```python
from build123d import *

# Parameters (mm, degrees)
SKETCH2_W           = 50
SKETCH2_H           = 50
BOSS_EXTRUDE1_DEPTH = 40
SKETCH4_R           = 3.25
CUT_EXTRUDE1_DEPTH  = 6
CUT_EXTRUDE2_DEPTH  = 34
SKETCH6_W           = 8
SKETCH6_H           = 13
CUT_EXTRUDE3_DEPTH  = 24
CUT_EXTRUDE4_DEPTH  = 7
SKETCH8_W           = 15
SKETCH8_H           = 20
CUT_EXTRUDE5_DEPTH  = 33
SKETCH8_3_W         = 5
SKETCH8_3_H         = 20
CUT_EXTRUDE6_DEPTH  = 24
CUT_EXTRUDE7_DEPTH  = 24
SKETCH7_W           = 3
SKETCH7_H           = 2
CUT_EXTRUDE8_DEPTH  = 10
SKETCH9_W           = 3
SKETCH9_H           = 3
CUT_EXTRUDE9_DEPTH  = 10
SKETCH12_W          = 50
SKETCH12_H          = 50
CUT_EXTRUDE10_DEPTH = 5
SKETCH16_W          = 5
SKETCH16_H          = 20
CUT_EXTRUDE11_DEPTH = 4
CUT_EXTRUDE12_DEPTH = 5
CUT_EXTRUDE13_DEPTH = 4
CUT_EXTRUDE14_DEPTH = 4
SKETCH11_W          = 5
SKETCH11_H          = 10
CUT_EXTRUDE15_DEPTH = 5
SKETCH20_R          = 6.5
CUT_EXTRUDE16_DEPTH = 29


with BuildPart() as part:
    # Sketch2 → Boss-Extrude1 (new body)
    with BuildSketch(Plane(origin=(0, 0, 0), x_dir=(1, 0, 0), z_dir=(0, 1, 0))):
        Rectangle(SKETCH2_W, SKETCH2_H)
    extrude(amount=-BOSS_EXTRUDE1_DEPTH)

    # Sketch4 → Cut-Extrude1 (cut)
    with BuildSketch(Plane(origin=(0, 0, 0), x_dir=(1, 0, 0), z_dir=(0, 1, 0))):
        with Locations(Location((15, -12.5, 0), (0, 0, 270))):
            Circle(SKETCH4_R)
        with Locations(Location((-15, -12.5, 0), (0, 0, 270))):
            Circle(SKETCH4_R)
        with Locations(Location((0, -12.5, 0), (0, 0, 270))):
            Circle(SKETCH4_R)
    extrude(amount=-CUT_EXTRUDE1_DEPTH, mode=Mode.SUBTRACT)

    # Sketch5 → Cut-Extrude2 (cut)
    with BuildSketch(Plane.XZ.offset(40)):
        Polygon((19, 12.5), (15, 12.5), (11, 12.5), (11, 6), (19, 6), align=None)
        Polygon((11, 12.5), (15, 12.5), (19, 12.5), (19, 19), (11, 19), align=None)
        Polygon((-11, 12.5), (-15, 12.5), (-19, 12.5), (-19, 6), (-11, 6), align=None)
        Polygon((-19, 12.5), (-15, 12.5), (-11, 12.5), (-11, 19), (-19, 19), align=None)
        Polygon((4, 12.5), (4, 6), (-4, 6), (-4, 19), (4, 19), align=None)
    extrude(amount=-CUT_EXTRUDE2_DEPTH, mode=Mode.SUBTRACT)

    # Sketch6 → Cut-Extrude3 (cut)
    with BuildSketch(Plane.XZ.offset(40)):
        Polygon((-20, 20), (-20, 3), (0, 3), (20, 3), (20, 20), align=None)
        with Locations((-15, 12.5)):
            Rectangle(SKETCH6_W, SKETCH6_H, mode=Mode.SUBTRACT)
        Polygon((4, 6), (0, 6), (-4, 6), (-4, 19), (4, 19), align=None, mode=Mode.SUBTRACT)
        with Locations((15, 12.5)):
            Rectangle(SKETCH6_W, SKETCH6_H, mode=Mode.SUBTRACT)
    extrude(amount=-CUT_EXTRUDE3_DEPTH, mode=Mode.SUBTRACT)

    # Sketch3 → Cut-Extrude4 (cut)
    with BuildSketch(Plane(origin=(0, 0, 0), x_dir=(1, 0, 0), z_dir=(0, 1, 0))):
        Polygon((19.5, 20), (19.5, 0), (-19.5, 0), (-19.5, 20), (0, 20), align=None)
    extrude(amount=-CUT_EXTRUDE4_DEPTH, mode=Mode.SUBTRACT)

    # Sketch8 → Cut-Extrude5 (cut)
    with BuildSketch(Plane.XZ.offset(40)):
        with Locations((-7.5, -10)):
            Rectangle(SKETCH8_W, SKETCH8_H)
        with Locations((7.5, -10)):
            Rectangle(SKETCH8_W, SKETCH8_H)
    extrude(amount=-CUT_EXTRUDE5_DEPTH, mode=Mode.SUBTRACT)

    # Sketch8_3 → Cut-Extrude6 (cut)
    with BuildSketch(Plane.XZ.offset(40)):
        with Locations((-17.5, -10)):
            Rectangle(SKETCH8_3_W, SKETCH8_3_H)
        with Locations((17.5, -10)):
            Rectangle(SKETCH8_3_W, SKETCH8_3_H)
    extrude(amount=-CUT_EXTRUDE6_DEPTH, mode=Mode.SUBTRACT)

    # Sketch8_4 → Cut-Extrude7 (cut)
    with BuildSketch(Plane.XZ.offset(40)):
        Polygon((20, 3), (-20, 3), (-20, 0), (-15, 0), (0, 0), (15, 0), (20, 0), align=None)
    extrude(amount=-CUT_EXTRUDE7_DEPTH, mode=Mode.SUBTRACT)

    # Sketch7 → Cut-Extrude8 (cut)
    with BuildSketch(Plane(origin=(0, -7, 0), x_dir=(1, 0, 0), z_dir=(0, 1, 0))):
        with Locations((-18, 19)):
            Rectangle(SKETCH7_W, SKETCH7_H)
        with Locations((-18, 1)):
            Rectangle(SKETCH7_W, SKETCH7_H)
        with Locations((18, 1)):
            Rectangle(SKETCH7_W, SKETCH7_H)
        with Locations((18, 19)):
            Rectangle(SKETCH7_W, SKETCH7_H)
    extrude(amount=-CUT_EXTRUDE8_DEPTH, mode=Mode.SUBTRACT)

    # Sketch9 → Cut-Extrude9 (cut)
    with BuildSketch(Plane.XZ.offset(40)):
        with Locations((-22.5, 22.5)):
            Rectangle(SKETCH9_W, SKETCH9_H)
        with Locations((-22.5, -22.5)):
            Rectangle(SKETCH9_W, SKETCH9_H)
        with Locations((22.5, -22.5)):
            Rectangle(SKETCH9_W, SKETCH9_H)
        with Locations((22.5, 22.5)):
            Rectangle(SKETCH9_W, SKETCH9_H)
    extrude(amount=-CUT_EXTRUDE9_DEPTH, mode=Mode.SUBTRACT)

    # Sketch12 → Cut-Extrude10 (cut)
    with BuildSketch(Plane.XZ.offset(40)):
        Rectangle(SKETCH12_W, SKETCH12_H)
    extrude(amount=-CUT_EXTRUDE10_DEPTH, mode=Mode.SUBTRACT)

    # Sketch16 → Cut-Extrude11 (cut)
    with BuildSketch(Plane.XZ.offset(16)):
        with Locations((17.5, -10)):
            Rectangle(SKETCH16_W, SKETCH16_H)
        with Locations((-17.5, -10)):
            Rectangle(SKETCH16_W, SKETCH16_H)
    extrude(amount=-CUT_EXTRUDE11_DEPTH, mode=Mode.SUBTRACT)

    # Sketch13 → Cut-Extrude12 (cut)
    with BuildSketch(Plane(origin=(0, 0, -25), x_dir=(-1, 0, 0), z_dir=(0, 0, -1))):
        Polygon((0, -16.279858657), (10, -16.279858657), (10, -22.279858657), (-10, -22.279858657), (-10, -16.279858657), align=None)
    extrude(amount=-CUT_EXTRUDE12_DEPTH, mode=Mode.SUBTRACT)

    # Sketch14 → Cut-Extrude13 (cut)
    with BuildSketch(Plane.XY.offset(-20)):
        Polygon((10, -19.279858657), (10, -12.279858657), (-20, -12.279858657), (-20, -36.279858657), (10, -36.279858657), align=None)
    extrude(amount=-CUT_EXTRUDE13_DEPTH, mode=Mode.SUBTRACT)

    # Sketch18 → Cut-Extrude14 (cut)
    with BuildSketch(Plane(origin=(-20, 0, 0), x_dir=(0, 0, -1), z_dir=(1, 0, 0))):
        Polygon((4, -29), (24, -29), (24, -12.279858657), (20, -12.279858657), (4, -12.279858657), align=None)
    extrude(amount=-CUT_EXTRUDE14_DEPTH, mode=Mode.SUBTRACT)

    # Sketch11 → Cut-Extrude15 (cut)
    with BuildSketch(Plane.XY.offset(25)):
        with Locations((2.5, -28.5)):
            Rectangle(SKETCH11_W, SKETCH11_H)
        with Locations((-2.5, -28.5)):
            Rectangle(SKETCH11_W, SKETCH11_H)
    extrude(amount=-CUT_EXTRUDE15_DEPTH, mode=Mode.SUBTRACT)

    # Sketch20 → Cut-Extrude16 (cut)
    with BuildSketch(Plane.XZ.offset(35)):
        with Locations((0, 12.5)):
            Circle(SKETCH20_R)
        with BuildLine():
            ThreePointArc((-20, 8.346688069), (-12.792059783, 6.38649037), (-8.5, 12.5))
            ThreePointArc((-8.5, 12.5), (-12.792059783, 18.61350963), (-20, 16.653311931))
            Line((-20, 16.653311931), (-20, 8.346688069))
        make_face()
        with BuildLine():
            Line((-20, 8.346688069), (-20, 16.653311931))
            ThreePointArc((-20, 16.653311931), (-21.5, 12.5), (-20, 8.346688069))
        make_face()
        with Locations((15, 12.5)):
            Circle(SKETCH20_R)
    extrude(amount=-CUT_EXTRUDE16_DEPTH, mode=Mode.SUBTRACT)


solid = part.part
```
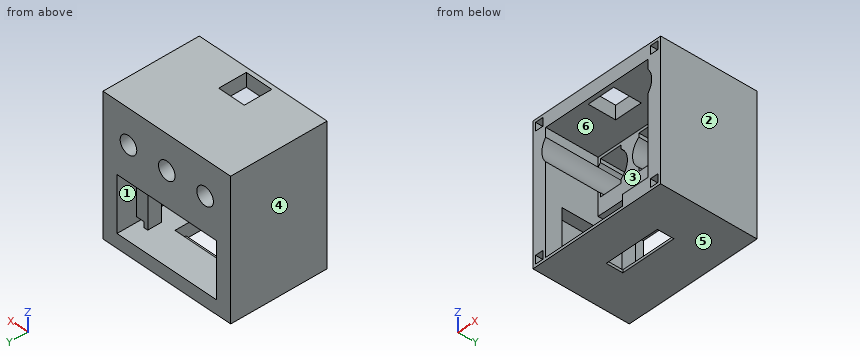
Input: part model. Units: mm. Frame: model coordinates. Face numbers are marked on the shaded views. A direction names the side the tool comes from. Give positions to 0.01 mm unless a question says otherwise; leave off trailing zeros. Order: outer loops, then holes, each group sorted by start corner. A loop starts at its lowest first (then second) coordinate and runs counter-clockwise, first axis right, second up. Notation, with made-up numbers: M 27,73.5 L 32,73.5 A32 ccw 32,107.5 Z; hole C 35,67.25 d6. An arc over 180 degrees is marked long. Return JSON: item names as keys, results as strings.
Item 1: First-contact query: P1, Ø5, axis at x = 15, z = 12.5, coming from the -Y side; P2, Ø12, axis at x = -1.5, z = 8, coming from the -Y side; P3, Ø8.5, axis at x = -15, z = 12.5, coming from the -Y side; P4, Ø10, axis at x = -11, z = -11.5, coming from the +Y side. Flat tips, straight axial feed; report the tip coordinate or a pass-through.
Solutions:
{"P1": "through", "P2": "y = -16", "P3": "y = -6", "P4": "y = -7"}
Item 2: Pull-direction query (X, two-part tool) for the marked faces 4, 5 and 6; classes: +X half, -X half, draft (parallel to the pull), parting line (faces both ways), or undercut.
Solutions:
{"face 4": "-X half", "face 5": "draft", "face 6": "undercut"}
Item 3: Access query for the marked faces 1, 2 and 3. Directions: +Z, -Z, +X, -X, +Y, -Y. A direction counts if a zero-diameter tool reaches every point of the face in a straight line with its end or side. Return the directions, or none.
Solutions:
{"face 1": "+Y", "face 2": "+Z, -Z, +X, +Y, -Y", "face 3": "-Y"}
Item 4: Cut plane A-A (x = 0). Return loops of the section in (y, z), then the cut area to 3 significant figures.
Solutions:
{"outline": "M -35,-25 L -22.28,-25 L -22.28,-24 L -35,-24 Z; M -35,20 L -33.5,20 L -33.5,25 L -35,25 Z; M -23.5,20 L -16,20 L -16,19 L -6,19 L -6,15.75 L 0,15.75 L 0,25 L -23.5,25 Z; M -16.28,-25 L 0,-25 L 0,-20 L -12.28,-20 L -12.28,-24 L -16.28,-24 Z; M -16,0 L 0,0 L 0,9.25 L -6,9.25 L -6,6 L -16,6 Z", "area": "354 mm^2"}
Item 5: Cut plane B-B (y = -3.5). Return loops of the section in (x, z), then the cut area to 3 significant figures.
Solutions:
{"outline": "M -25,-25 L 25,-25 L 25,25 L -25,25 Z; hole M -19.5,-20 L 19.5,-20 L 19.5,0 L -19.5,0 Z; hole C -15,12.5 d6.5; hole C 0,12.5 d6.5; hole C 15,12.5 d6.5", "area": "1,620 mm^2"}
Item 6: Ray query, probe 1 along X at (y, z) = (-1.9, 12.5); probe 2 along X at (y, z) = (-17.5, 6.5); probe 3 along Z at (x, y) = (-20.5, -12.5). Return the intervals inside material, ascending.
Solutions:
{"probe 1": "-25 to -18.25, -11.75 to -3.25, 3.25 to 11.75, 18.25 to 25", "probe 2": "-25 to -20, 20 to 25", "probe 3": "-25 to -24, -4 to 9.04, 15.96 to 25"}
Item 7: Cut plane C-C (z = 2.5). Return loops of the section in (x, y).
Solutions:
{"outline": "M -25,-35 L -20,-35 L -20,-16 L 20,-16 L 20,-35 L 25,-35 L 25,0 L -25,0 Z"}
Item 8: Cut plane D-D (y = -17.5). Return loops of the section in (x, z).
Solutions:
{"outline": "M -25,-25 L -10,-25 L -10,-24 L -24,-24 L -24,-4 L -20,-4 L -20,8.35 A6.5 cw -20,16.65 L -20,20 L 20,20 L 20,16.65 A6.5 cw 20,8.35 L 20,-20 L 10,-20 L 10,-25 L 25,-25 L 25,25 L -25,25 Z"}
